Answer from the drawing. Dimensions are ordinates in mm from the lowest x, y and z of the part. Coordinates: 2 decimals unless noted, no trailing zeros. Write each loop counter-clockwise with the first axis right and the second up, starting at its lowest first coordinate (ties: lowest second). Pieces come first, ordered by that corner, then holes. Notation, with made-up numbers: (75.5, 11) - (84.5, 11) arc R30 ccw to (84.5, 48) - close; hole circle Ø8 at (-40, -2). An arc over 180 degrees is marked (long way). Use a Markdown table: item, result.
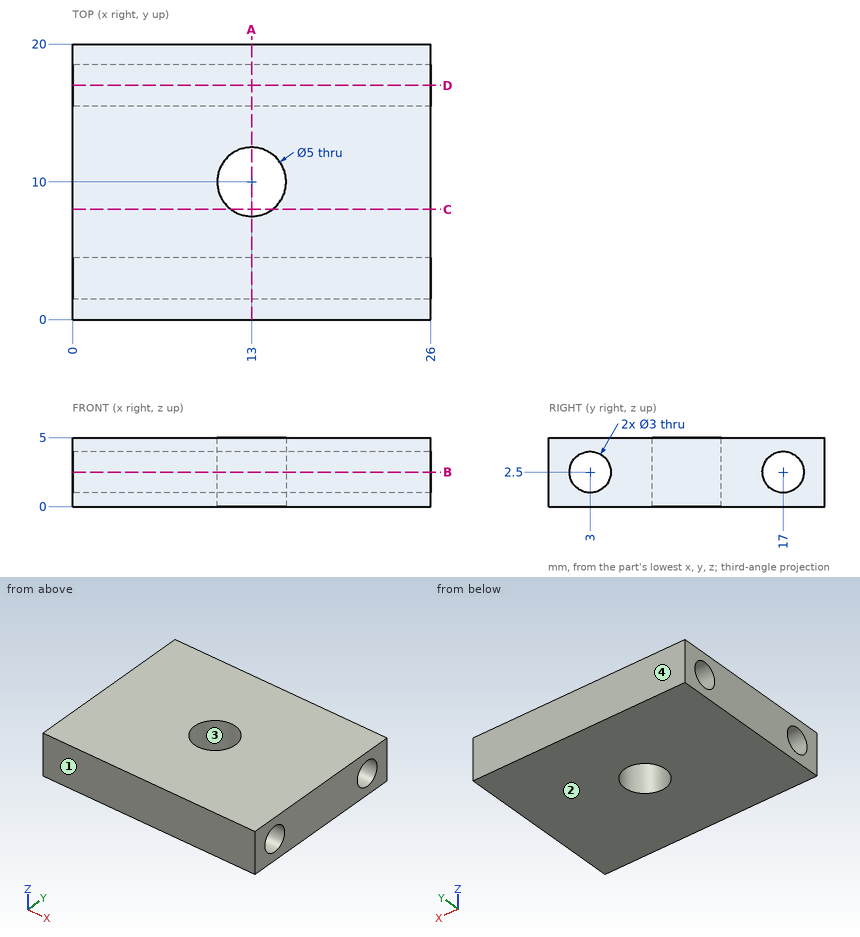
(1) Straight lines are drawn through the part: L1, parallel to Y at x = 7.25, z = 2.6; L2, parallel to Z at x = 8.5, y = 3; L3, parallel to Y at x = 11, z = 1.55. For each, find the intervals that lie inside material, in ascending order.
Report:
| item | result |
|---|---|
| L1 | y = 0 to 1.5, 4.5 to 15.5, 18.5 to 20 |
| L2 | z = 0 to 1, 4 to 5 |
| L3 | y = 0 to 1.84, 4.16 to 8.5, 11.5 to 15.84, 18.16 to 20 |
(2) A cutting plane is placed at D-D, the plane y = 17. Write down the section's boundary in (x, z).
Report:
| item | result |
|---|---|
| outline | (0, 0) - (26, 0) - (26, 1) - (0, 1) - close; (0, 4) - (26, 4) - (26, 5) - (0, 5) - close |
(3) A cutting plane is placed at C-C, the plane y = 8. Write down the section's boundary in (x, z).
Report:
| item | result |
|---|---|
| outline | (0, 0) - (11.5, 0) - (11.5, 5) - (0, 5) - close; (14.5, 0) - (26, 0) - (26, 5) - (14.5, 5) - close |
(4) A cutting plane is placed at B-B, the plane z = 2.5. Write down the section's boundary in (x, y).
Report:
| item | result |
|---|---|
| outline | (0, 0) - (26, 0) - (26, 1.5) - (0, 1.5) - close; (0, 4.5) - (26, 4.5) - (26, 15.5) - (0, 15.5) - close; (0, 18.5) - (26, 18.5) - (26, 20) - (0, 20) - close; hole circle Ø5 at (13, 10) |
(5) The mould has two halves that part along Y. Classify the marked faces 1, 2, 3 and 4: pulls with the +Y half, pulls with the -Y half, needs draft (parallel to the pull), parting line crosses it, or undercut.
Report:
| item | result |
|---|---|
| face 1 | pulls with the -Y half |
| face 2 | needs draft |
| face 3 | undercut |
| face 4 | pulls with the +Y half |
(6) A cutting plane is placed at A-A, the plane x = 13. Write down the section's boundary in (y, z).
Report:
| item | result |
|---|---|
| outline | (0, 0) - (7.5, 0) - (7.5, 5) - (0, 5) - close; (12.5, 0) - (20, 0) - (20, 5) - (12.5, 5) - close; hole circle Ø3 at (3, 2.5); hole circle Ø3 at (17, 2.5) |
